Model file for the job. Use its own axes, mm. A direction names the side the tool comes from. Round coordinates to 2 decimals unless told otherwise and drop trailing zeros. Order: outer loops, then holes, each group sorted by start corner. A loop starts at its lowest first (then second) coordinate and runs counter-clockwise, first axis right, second up. Notation, with made-up numbers: (26.25, 66) - (38.25, 66) arc R29 ccw to (38.25, 92) - close; hole circle Ø2 at (31.5, 55.5). An arc over 180 degrees is marked (long way). Write item = value, one per line.
```python
from build123d import *

# Parameters (mm, degrees)
ESQUISSE1_W        = 24.82
ESQUISSE1_H        = 23.3
ESQUISSE1_R        = 0.55
BOSS_EXTRU_1_DEPTH = 1.64
ESQUISSE2_W        = 18
ESQUISSE2_H        = 15.84
BOSS_EXTRU_2_DEPTH = 2.46
ESQUISSE3_W        = 7.36
ESQUISSE3_H        = 4.24
BOSS_EXTRU_3_DEPTH = 2.9
ESQUISSE4_W        = 4.5
ESQUISSE4_H        = 1.4
BOSS_EXTRU_4_DEPTH = 1.4


with BuildPart() as part:
    # Esquisse1 → Boss.-Extru.1 (new body)
    with BuildSketch(Plane(origin=(0, 0, 0), x_dir=(1, 0, 0), z_dir=(0, 1, 0))):
        with Locations((12.41, 11.65)):
            Rectangle(ESQUISSE1_W, ESQUISSE1_H)
        with Locations(Location((1.85, 5.55, 0), (0, 0, 270))):
            Circle(ESQUISSE1_R, mode=Mode.SUBTRACT)
        with Locations(Location((23.37, 3.05, 0), (0, 0, 270))):
            Circle(ESQUISSE1_R, mode=Mode.SUBTRACT)
        with Locations(Location((1.85, 8.09, 0), (0, 0, 270))):
            Circle(ESQUISSE1_R, mode=Mode.SUBTRACT)
        with Locations(Location((23.37, 5.59, 0), (0, 0, 270))):
            Circle(ESQUISSE1_R, mode=Mode.SUBTRACT)
        with Locations(Location((1.85, 10.63, 0), (0, 0, 270))):
            Circle(ESQUISSE1_R, mode=Mode.SUBTRACT)
        with Locations(Location((23.37, 8.13, 0), (0, 0, 270))):
            Circle(ESQUISSE1_R, mode=Mode.SUBTRACT)
        with Locations(Location((1.85, 13.17, 0), (0, 0, 270))):
            Circle(ESQUISSE1_R, mode=Mode.SUBTRACT)
        with Locations(Location((23.37, 10.67, 0), (0, 0, 270))):
            Circle(ESQUISSE1_R, mode=Mode.SUBTRACT)
        with Locations(Location((1.85, 15.71, 0), (0, 0, 270))):
            Circle(ESQUISSE1_R, mode=Mode.SUBTRACT)
        with Locations(Location((23.37, 13.21, 0), (0, 0, 270))):
            Circle(ESQUISSE1_R, mode=Mode.SUBTRACT)
        with Locations(Location((1.85, 18.25, 0), (0, 0, 270))):
            Circle(ESQUISSE1_R, mode=Mode.SUBTRACT)
        with Locations(Location((23.37, 15.75, 0), (0, 0, 270))):
            Circle(ESQUISSE1_R, mode=Mode.SUBTRACT)
    extrude(amount=BOSS_EXTRU_1_DEPTH)

    # Esquisse2 → Boss.-Extru.2 (add)
    with BuildSketch(Plane(origin=(0, 1.64, 0), x_dir=(1, 0, 0), z_dir=(0, 1, 0))):
        with Locations((12.8, 9.02)):
            Rectangle(ESQUISSE2_W, ESQUISSE2_H)
    extrude(amount=BOSS_EXTRU_2_DEPTH)

    # Esquisse3 → Boss.-Extru.3 (add)
    with BuildSketch(Plane(origin=(0, 1.64, 0), x_dir=(1, 0, 0), z_dir=(0, 1, 0))):
        with Locations((9.281405269, 19.914341586)):
            Rectangle(ESQUISSE3_W, ESQUISSE3_H)
    extrude(amount=BOSS_EXTRU_3_DEPTH)

    # Esquisse4 → Boss.-Extru.4 (add)
    with BuildSketch(Plane.XZ):
        Polygon((15.72, -7.6), (4.92, -7.6), (4.92, -23.3), (20.22, -23.3), (20.22, -7.6), align=None)
        with Locations((17.97, -6.9)):
            Rectangle(ESQUISSE4_W, ESQUISSE4_H)
    extrude(amount=BOSS_EXTRU_4_DEPTH)


solid = part.part
```
1) Cut at C-C (z = -12). Write the cut outline in (x, y).
Conclusion:
outline = (0, 0) - (4.92, 0) - (4.92, -1.4) - (20.22, -1.4) - (20.22, 0) - (24.82, 0) - (24.82, 1.64) - (21.8, 1.64) - (21.8, 4.1) - (3.8, 4.1) - (3.8, 1.64) - (0, 1.64) - close
2) Cut at A-A (y = 3.5). Write the cut outline in (x, z), and give its area (3 significant figures).
Conclusion:
outline = (3.8, -16.94) - (21.8, -16.94) - (21.8, -1.1) - (3.8, -1.1) - close; (5.6, -22.03) - (12.96, -22.03) - (12.96, -17.79) - (5.6, -17.79) - close
area = 316 mm^2
3) Mould opens along Z. For faces 4 (the face through (9, 3, -17.794)), 5 (the face through (20.22, -1, -15)), 6 (the face through (10, -1, -7.6)) say: +Z half, -Z half, draft (parallel to the pull), parting line (faces both ways), or undercut.
Conclusion:
face_4 = undercut
face_5 = draft
face_6 = +Z half
4) Cut at D-D (x = 9). Write the cut outline in (y, z), and give its area (3 significant figures).
Conclusion:
outline = (-1.4, -23.3) - (1.64, -23.3) - (1.64, -22.03) - (4.54, -22.03) - (4.54, -17.79) - (1.64, -17.79) - (1.64, -16.94) - (4.1, -16.94) - (4.1, -1.1) - (1.64, -1.1) - (1.64, 0) - (0, 0) - (0, -7.6) - (-1.4, -7.6) - close
area = 111 mm^2
5) 3-axis set-ups, long thin cutter, end or side, ignore diameter. For faces 1 (the face through (13, 4.1, -9)), 2 (the face through (4.92, -1, -15)), 3 (the face through (12.961, 3, -20)): which of +Z, -Z, +X, -X, +Y, -Y reach the whole face in a straight line?
Conclusion:
face_1 = +Z, +X, -X, +Y
face_2 = +Z, -Z, -X, -Y
face_3 = -Z, +X, +Y
6) Wall check: line 1 along X through (y, z) = (0.95, -10.63); line 2 along Z through (x, y) = (6.75, 2.05); line 3 along Y through (x, z) = (10, -5). Give the ranges that are in metal, low to high.
Conclusion:
line_1 = 0 to 1.3, 2.4 to 22.82, 23.92 to 24.82
line_2 = -22.03 to -17.79, -16.94 to -1.1
line_3 = 0 to 4.1
7) Cut at B-B (y = 0.45). Give the number of separate pieces and of enclosed holes in the cut face, and give its area (3 significant figures).
Conclusion:
separate_pieces = 1
enclosed_holes = 12
area = 567 mm^2
8) Flat gauge pins, fed straight in: pin 1 Ø0.7 at (x, z) = (1.85, -8.09) entering from -Y; pin 2 Ø1.4 at (x, z) = (23.37, -13.21) entering from -Y; pin 3 Ø0.7 at (y, z) = (3, -5.5) entering from +X; pin 4 Ø5 at (x, z) = (9, -4) entering from +Y. Where does each tip first touch, or does it go through?
Conclusion:
pin_1 = through
pin_2 = 0
pin_3 = 21.8
pin_4 = 4.1
